Here's the drawing with two shaded views (mm, measured from the low corner). I have some questions. A direction names the side the tool comes from. Round coordinates to 2 decimals unless told otherwise and drop trailing zeros. Loops run counter-clockwise (first coordinate to the right, second up) from the corner with the lowest first, then second, coordinate; pieces in that order, holes last. Notation, with made-up numbers: (73.5, 74.5) -> (88.5, 74.5) arc R20 ccw to (88.5, 108.5) -> close; hole circle Ø9 at (83, -28). An arc over 180 degrees is marked (long way). Write each question's results on one line, items separated by ' | '. Start each with the question number.
1) Which directions (+Z, -Z, +X, -X, +Y, -Y) give clear straight access to the entire face, cutting with the end or side of a thin tool? Please do the marked faces 5 and 6.
2) Imagine slicing it at A-A, the plane y = 2.65. List the corners of the cut face in (x, z) for me (1 decimal).
3) Imagine slicing it at C-C, the plane x = 2. List the corners of the cut face in (y, z) for me, plus the area to 3 significant figures.
4) If I drill on probe 1 along Z at (x, y) = (2.75, 2.5); probe 2 along Z at (x, y) = (4, 0.25) (1 decimal); probe 3 along X at (y, z) = (0.2, 3.1) (1 decimal), over which ranges is the centre line in solid material (lowest first)?
5) For P1, Ø3, axis at x = 3.18, z = 2.75, coming from the +Y side; P2, Ø1, axis at x = 1.5, y = 1.5, coming from the -Z side; P3, Ø2, axis at y = 2, z = 1, coming from the -X side (1 decimal), each with a flat end and sliding along its axis, tell me the tip position at first contact or that it passes through.
6) Imagine slicing it at B-B, the plane z = 1.8. List the corners of the cut face in (x, y) for me.
7) Imagine slicing it at D-D, the plane z = 4.3. List the corners of the cut face in (x, y) for me (1 decimal), plus the area to 3 significant figures.
8) We'd pull the mould along X, two halves only. Please class the marked faces 1, 2, 3 and 4: pulls with the +X half, pulls with the -X half, needs draft (parallel to the pull), parting line crosses it, or undercut.
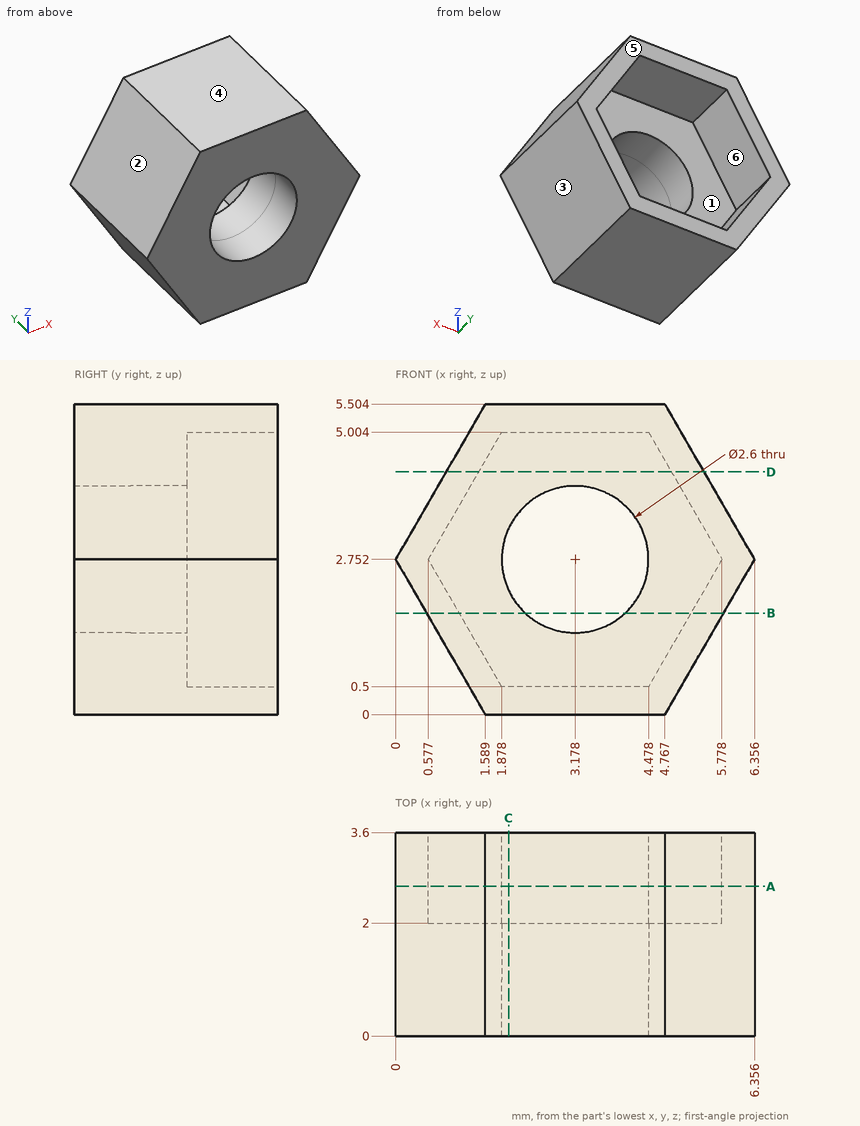
Checked values:
1) face 5: +Z, -Z, +X, -X, +Y | face 6: +Y
2) outline: (0, 2.8) -> (1.6, 0) -> (4.8, 0) -> (6.4, 2.8) -> (4.8, 5.5) -> (1.6, 5.5) -> close; hole (0.6, 2.8) -> (1.9, 0.5) -> (4.5, 0.5) -> (5.8, 2.8) -> (4.5, 5) -> (1.9, 5) -> close
3) outline: (0, 0) -> (3.6, 0) -> (3.6, 0.5) -> (2, 0.5) -> (2, 2.2) -> (0, 2.2) -> close; (0, 3.3) -> (2, 3.3) -> (2, 5) -> (3.6, 5) -> (3.6, 5.5) -> (0, 5.5) -> close | area: 10.4 mm^2
4) probe 1: 0 to 0.5, 5 to 5.5 | probe 2: 0 to 1.7, 3.8 to 5.5 | probe 3: 0.2 to 1.9, 4.4 to 6.2
5) P1: y = 2 | P2: z = 0 | P3: x = 0.4
6) outline: (0.55, 0) -> (2.29, 0) -> (2.29, 2) -> (1.13, 2) -> (1.13, 3.6) -> (0.55, 3.6) -> close; (4.06, 0) -> (5.81, 0) -> (5.81, 3.6) -> (5.23, 3.6) -> (5.23, 2) -> (4.06, 2) -> close
7) outline: (0.9, 0) -> (5.5, 0) -> (5.5, 3.6) -> (4.9, 3.6) -> (4.9, 2) -> (1.5, 2) -> (1.5, 3.6) -> (0.9, 3.6) -> close | area: 11.0 mm^2
8) face 1: undercut | face 2: pulls with the -X half | face 3: pulls with the +X half | face 4: needs draft
